Model file for the job. Use its own axes, mm. Face numbers are marked on the shaded views. A direction names the side the tool comes from. Coordinates: 2 decimals unless noted, no trailing zeros. Loops run counter-clockwise (first coordinate to the right, second up) from the corner with the lowest first, then second, coordinate; pieces in that order, holes last. Notation, with made-up numbers: (43.5, -36) - (73.5, -36) arc R8 ccw to (73.5, -29) - close; hole circle Ø3 at (-10.5, 45). An arc over 180 degrees is marked (long way). Write each question's results on one line, items separated by ' | '. Start each with the question number.
```python
from build123d import *

# Parameters (mm, degrees)
BOSS_EXTRUDE1_DEPTH = 2
SKETCH2_R           = 8.5
BOSS_EXTRUDE3_DEPTH = 31
SKETCH3_R           = 4.45
CUT_EXTRUDE1_DEPTH  = 33
FILLET1_R           = 1
SKETCH4_W           = 11.502222151
SKETCH4_H           = 31
CUT_EXTRUDE2_DEPTH  = 20
FILLET2_R           = 10
FILLET3_R           = 2.5


with BuildPart() as part:
    # Sketch1 → Boss-Extrude1 (new body)
    with BuildSketch(Plane(origin=(0, 0, 0), x_dir=(1, 0, 0), z_dir=(0, 1, 0))):
        Polygon((0, 15.5), (15.5, 15.5), (15.5, -15.5), (-15.5, -15.5), (-15.5, 15.5), align=None)
    extrude(amount=BOSS_EXTRUDE1_DEPTH)

    # Sketch2 → Boss-Extrude3 (add)
    with BuildSketch(Plane(origin=(15.5, 0, 0), x_dir=(0, 0, -1), z_dir=(1, 0, 0))):
        with Locations((0, 8.5)):
            Circle(SKETCH2_R)
    extrude(amount=-BOSS_EXTRUDE3_DEPTH)

    # Sketch3 → Cut-Extrude1 (cut)
    with BuildSketch(Plane.ZY.offset(15.5)):
        with Locations((0, 13.5)):
            Circle(SKETCH3_R)
    extrude(amount=-CUT_EXTRUDE1_DEPTH, mode=Mode.SUBTRACT)

    # Fillet1
    fillet1_edges = [part.edges().sort_by_distance(p)[0] for p in [
        (0, 16.24475, -3.502691456),
        (0, 16.24475, 3.502691456),
    ]]
    fillet(fillet1_edges, radius=FILLET1_R)

    # Sketch4 → Cut-Extrude2 (cut)
    with BuildSketch(Plane(origin=(0, 2, 0), x_dir=(1, 0, 0), z_dir=(0, 1, 0))):
        with Locations((0.251111076, 0)):
            Rectangle(SKETCH4_W, SKETCH4_H)
    extrude(amount=CUT_EXTRUDE2_DEPTH, mode=Mode.SUBTRACT)

    # Fillet2
    fillet2_edges = [part.edges().sort_by_distance(p)[0] for p in [
        (15.5, 1, -15.5),
        (15.5, 1, 15.5),
        (-15.5, 1, 15.5),
        (-15.5, 1, -15.5),
    ]]
    fillet(fillet2_edges, radius=FILLET2_R)

    # Fillet3
    fillet3_edges = [part.edges().sort_by_distance(p)[0] for p in [
        (-5.5, 2, 0),
        (6.002222151, 2, 0),
    ]]
    fillet(fillet3_edges, radius=FILLET3_R)


solid = part.part
```
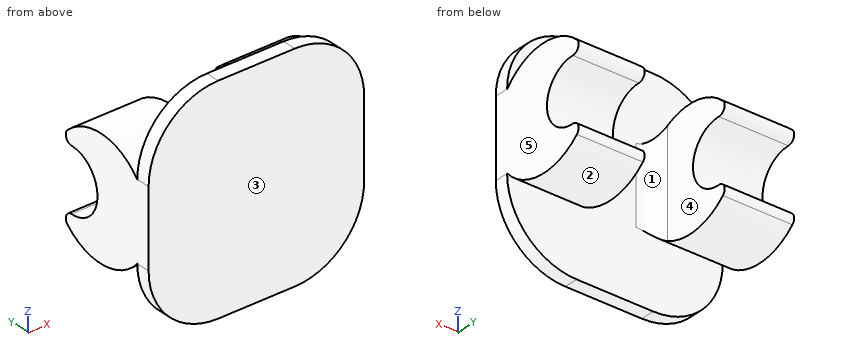
Q1. Drill centre lines: L1, parallel to X at y = 10.25, z = 6.5; L2, parallel to Y at x = -3, z = -12; L3, parallel to Z at x = -9, y = 8.25. Where is each one in solid material? Low to high. Write a range as from..to.
Q2. Cut at D-D (x = 5). List the corners of the cut face in (y, z).
Q3. Cut at C-C (z = 0). List the corners of the cut face in (x, y), and give its area (3 significant figures).
Q4. Pin check, flat tips, straight feed: pin 1 (5 mm diameter, centred on x = 9, z = -0.5, fed in from +Y); pin 2 (6 mm diameter, centred on x = 8, y = 9, fed in from +Z). Stop position of each tip, or through.
Q5. Cut at B-B (y = 2.5). List the corners of the cut face in (x, z).
Q6. Cut at A-A (z = -8). List the corners of the cut face in (x, y).
Q7. Which spindle directions (+Z, -Z, +X, -X, +Y, -Y) get a long thin tool onto all of the face, cutting with end or side? Do the marked faces 4 and 5. Say none if no direction does.
Q8. Mould opens along Y. For the marked faces 1, 2 and 3 say: +Y half, -Y half, draft (parallel to the pull), parting line (faces both ways), or undercut.
Check result:
1) L1: -15.5..-5.5, 6..15.5 | L2: 0..2 | L3: -8.5..8.5
2) outline: (0, -15.5) - (2, -15.5) - (2, -5.48) arc R8.5 ccw to (2.5, -6.02) - (2.5, 6.02) arc R8.5 ccw to (2, 5.48) - (2, 15.5) - (0, 15.5) - close
3) outline: (-15.5, 0) - (15.5, 0) - (15.5, 9.05) - (6, 9.05) - (6, 4.5) arc R2.5 cw to (3.5, 2) - (-3, 2) arc R2.5 cw to (-5.5, 4.5) - (-5.5, 9.05) - (-15.5, 9.05) - close | area: 202 mm²
4) pin 1: y = 10.21 | pin 2: z = 8.5
5) outline: (-15.5, -6.02) - (-4.5, -6.02) - (-4.5, 6.02) - (-15.5, 6.02) - close; (5, -6.02) - (15.5, -6.02) - (15.5, 6.02) - (5, 6.02) - close
6) outline: (-15.5, 5.63) - (-5.5, 5.63) - (-5.5, 11.37) - (-15.5, 11.37) - close; (-15.18, 0) - (15.18, 0) - (15.18, 2) - (-15.18, 2) - close; (6, 5.63) - (15.5, 5.63) - (15.5, 11.37) - (6, 11.37) - close
7) face 4: +Z, -Z, +Y | face 5: +Z, -Z, +X, +Y, -Y
8) face 1: +Y half | face 2: undercut | face 3: -Y half
